Read the model definition and answer for the solid it produces. Units are mm, in the model's axes. A direction names the side the tool comes from. Coordinates: 2 decimals unless noted, no trailing zeros. Write each loop counter-clockwise with the first axis right and the second up, starting at its lowest first coordinate (ties: lowest second). Pieces come first, ordered by that corner, then holes.
Item 1: Each of these flat-tipped pins is pushed along its axis until it touches: P1, Ø10, axis at x = -9.5, y = -11.5, coming from the +Z side; P2, Ø1, axis at x = 25.5, z = -1, coming from the +Y side; P3, Ø10, axis at y = -1, z = 30.5, coming from the +X side; P4, Ø5, axis at y = -3, z = 1, coming from the -X side. Where does it stop, or does it pass through?
Item 2: Determine the mould class of faces 4 (the face through (-3.638, 16.384, 24.79)), 5 (the face through (4, 11, 46)), 6 (the face through (13.935, -4.388, 24.79)) for opening direction Y: released by +Y, released by -Y, zero draft, split by the parting line, or undercut.
Item 3: Section A-A (x = 0) is taken. Give the vertices of the cut face in (y, z) (3 decimals).
Item 4: Straight lines are drawn through the part: probe 1 along Y at (x, z) = (0, -9.25); probe 2 along Y at (x, z) = (-1, 3.5); probe 3 along X at (y, z) = (19, 8). For each, find the intervals that lie inside material, in ascending order.
Item 5: Section C-C (z = 24) is taken. Give the vertices of the cut face in (x, y), then the cut area to 3 significant figures.
Item 6: A tool of negligible diameter and unlimited length cuts with its end or side. For faces 1 (the face through (-29.97, 1.32, -8.87)), 2 (the face through (-9.03, 6.92, 37.89)), 3 (the face through (-2.899, 13.057, 37.888)), from which of +Z, -Z, +X, -X, +Y, -Y can it reach the whole face along a straight path? Write none if from no direction.
Item 7: Section B-B (z = 33.5) is taken. Give the vertices of the cut face in (x, y) (3 decimals).
Autodesk Fusion 360 part; units mm, degrees
sketch "Boceto1" plane through (0, 0, 0) normal (0, 0, 1) x (1, 0, 0)
  circle A0 centre (0, 0) radius 30
  circle A1 centre (0, 0) radius 33
  dimension "d1" = 60
  dimension "d10" = 3
ref_plane "PlanoDeObra1" through (0, 0, 30) normal (0, 0, 1) x (1, 0, 0)
sketch "Boceto2" plane through (0, 0, 30) normal (0, 0, 1) x (1, 0, 0)
  circle A0 centre (0, 0) radius 13.375
  circle A1 centre (0, 0) radius 11.375
  dimension "d4" = 26.75
  dimension "d5" = -2
loft "Solevación1" add profiles "Boceto2", "Boceto1" section 1 section 2
loft "Solevación2" cut profiles "Boceto2", "Boceto1" section 1 contours A1 section 2 contours A0
extrude "Extruir1" add sketch "Boceto2" along normal blind 16
extrude "Extruir2" add sketch "Boceto1" against normal blind 18
sketch "Boceto3" plane through (0, 0, 0) normal (0, 0, 1) x (1, 0, 0)
Established:
1. P1: stops at z = 46
1. P2: stops at y = 21.54
1. P3: stops at x = 16.3
1. P4: stops at x = -32.99
2. face 4: split by the parting line
2. face 5: zero draft
2. face 6: undercut
3. outline: (-33, -18) - (-30, -18) - (-30, 0) - (-11.375, 30) - (-11.375, 46) - (-13.375, 46) - (-13.375, 30) - (-33, 0) - close; (11.375, 30) - (30, 0) - (30, -18) - (33, -18) - (33, 0) - (13.375, 30) - (13.375, 46) - (11.375, 46) - close
4. probe 1: y = -33 to -30, 30 to 33
4. probe 2: y = -30.69 to -27.81, 27.81 to 30.69
4. probe 3: x = -20.25 to -16.3, 16.3 to 20.25
5. outline: circle Ø34.6 at (0, 0); hole circle Ø30.2 at (0, 0)
5. area: 224 mm2
6. face 1: -Z
6. face 2: +Z, -Z
6. face 3: +Z
7. outline: circle Ø26.75 at (0, 0); hole circle Ø22.75 at (0, 0)
